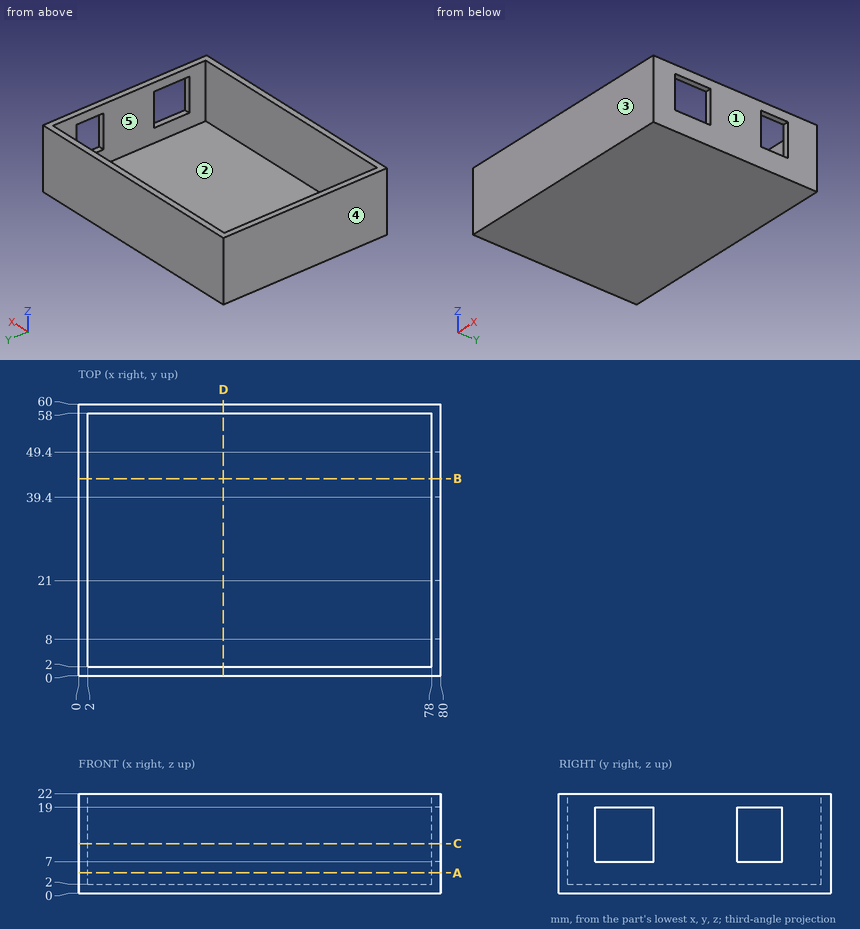
The drawing under review shows one solid part. Ordinate dimensions are in mm from its lowest x, y, z. A direction names the side the tool comes from. Coordinates: 2 decimals unless noted, no trailing zeros. Order: outer loops, then holes, each group sorted by start corner. A loop starts at its lowest first (then second) coordinate and runs counter-clockwise, first axis right, second up. Notation, with made-up numbers: (30, 30.5) -> (61, 30.5) arc R29 cw to (61, 65.5) -> close; hole circle Ø1 at (30, 47). An arc over 180 degrees is marked (long way). Use CSV: the item, a comma, the result in double quotes. Start each with the question number.
Item 1: Wall thickness on probe 1 along X at (y, z) = (46, 3); probe 2 along Y at (x, z) = (51, 4.5); probe 3 along Z at (x, y) = (7.5, 29): over which ranges is each line inside the solid? List them lowest first.
Item 2: We need section C-C, the plane z = 11. Give the boundary of the cut face in (x, y).
Item 3: We need section D-D, the plane x = 32. Give the boundary of the cut face in (y, z), then the cut area to 3 significant figures.
Item 4: Draft analysis for pull direction Y (two halves, no side actions). For the marked faces 3, 4 and 5, state which applies: pulls with the +Y half, pulls with the -Y half, needs draft (parallel to the pull), parting line crosses it, or undercut.
Item 5: We need section B-B, the plane y = 43.5. Give the boundary of the cut face in (x, z), then the cut area to 3 significant figures.
Item 6: Insertion check: pin 1 (1 mm diameter, centred on x = 39, y = 20, fed in from +Z). The pin has a flat end and moves straight along its axis. Give the tip position at first contact, or say it passes through.
Item 7: We need section A-A, the plane z = 4.5. Give the boundary of the cut face in (x, y).
Item 8: For the marked faces 1 and 2, list the 3-axis set-ups (+Z, -Z, +X, -X, +Y, -Y) from which the entire face can be reached by the end or side of a thin tool; tool diameter is ignored.
Derived:
1,probe 1,"x = 0 to 2, 78 to 80"
1,probe 2,"y = 0 to 2, 58 to 60"
1,probe 3,"z = 0 to 2"
2,outline,"(0, 0) -> (80, 0) -> (80, 8) -> (78, 8) -> (78, 2) -> (2, 2) -> (2, 58) -> (78, 58) -> (78, 49.4) -> (80, 49.4) -> (80, 60) -> (0, 60) -> close; (78, 21) -> (80, 21) -> (80, 39.4) -> (78, 39.4) -> close"
3,outline,"(0, 0) -> (60, 0) -> (60, 22) -> (58, 22) -> (58, 2) -> (2, 2) -> (2, 22) -> (0, 22) -> close"
3,area,"200 mm^2"
4,face 3,"pulls with the -Y half"
4,face 4,"needs draft"
4,face 5,"undercut"
5,outline,"(0, 0) -> (80, 0) -> (80, 7) -> (78, 7) -> (78, 2) -> (2, 2) -> (2, 22) -> (0, 22) -> close; (78, 19) -> (80, 19) -> (80, 22) -> (78, 22) -> close"
5,area,"216 mm^2"
6,pin 1,"stops at z = 2"
7,outline,"(0, 0) -> (80, 0) -> (80, 60) -> (0, 60) -> close; hole (2, 2) -> (78, 2) -> (78, 58) -> (2, 58) -> close"
8,face 1,"+Z, -Z, +X, +Y, -Y"
8,face 2,"+Z"
